from build123d import *

# Parameters (mm, degrees)
SKETCH1_W           = 160
SKETCH1_H           = 90
SKETCH1_R           = 20
SKETCH1_R_2         = 1.5
SKETCH1_W_2         = 10
SKETCH1_H_2         = 3
BOSS_EXTRUDE1_DEPTH = 3


with BuildPart() as part:
    # Sketch1 → Boss-Extrude1 (new body)
    with BuildSketch(Plane(origin=(0, 0, 0), x_dir=(1, 0, 0), z_dir=(0, 1, 0))):
        with Locations((-80, 45)):
            Rectangle(SKETCH1_W, SKETCH1_H)
        with Locations(Location((-40, 50, 0), (0, 0, 270))):
            Circle(SKETCH1_R, mode=Mode.SUBTRACT)
        with Locations(Location((-105, 4, 0), (0, 0, 270))):
            Circle(SKETCH1_R_2, mode=Mode.SUBTRACT)
        with Locations(Location((-45, 4, 0), (0, 0, 270))):
            Circle(SKETCH1_R_2, mode=Mode.SUBTRACT)
        with Locations(Location((-105, 86, 0), (0, 0, 90))):
            Circle(SKETCH1_R_2, mode=Mode.SUBTRACT)
        with Locations(Location((-45, 86, 0), (0, 0, 90))):
            Circle(SKETCH1_R_2, mode=Mode.SUBTRACT)
        with Locations(Location((-140, 67, 0), (0, 0, 270))):
            Circle(SKETCH1_R_2, mode=Mode.SUBTRACT)
        with Locations(Location((-140, 44, 0), (0, 0, 90))):
            Circle(SKETCH1_R_2, mode=Mode.SUBTRACT)
        with Locations(Location((-140, 22, 0), (0, 0, 270))):
            Circle(SKETCH1_R_2, mode=Mode.SUBTRACT)
        Polygon((-118, 68.4), (-118, 31.8), (-90, 31.8), (-80, 41.8), (-68, 41.8), (-61, 45), (-61, 55), (-68, 58.4), (-80, 58.4), (-90, 68.4), align=None, mode=Mode.SUBTRACT)
        with Locations((-135, 84.5)):
            Rectangle(SKETCH1_W_2, SKETCH1_H_2, mode=Mode.SUBTRACT)
        with Locations((-135, 5.5)):
            Rectangle(SKETCH1_W_2, SKETCH1_H_2, mode=Mode.SUBTRACT)
        with Locations((-75, 5.5)):
            Rectangle(SKETCH1_W_2, SKETCH1_H_2, mode=Mode.SUBTRACT)
        with Locations((-75, 84.5)):
            Rectangle(SKETCH1_W_2, SKETCH1_H_2, mode=Mode.SUBTRACT)
        with Locations((-15, 5.5)):
            Rectangle(SKETCH1_W_2, SKETCH1_H_2, mode=Mode.SUBTRACT)
        with Locations((-15, 84.5)):
            Rectangle(SKETCH1_W_2, SKETCH1_H_2, mode=Mode.SUBTRACT)
        with Locations((-151, 67)):
            Rectangle(SKETCH1_W_2, SKETCH1_H_2, mode=Mode.SUBTRACT)
        with Locations((-129, 67)):
            Rectangle(SKETCH1_W_2, SKETCH1_H_2, mode=Mode.SUBTRACT)
        with Locations((-129, 44)):
            Rectangle(SKETCH1_W_2, SKETCH1_H_2, mode=Mode.SUBTRACT)
        with Locations((-151, 44)):
            Rectangle(SKETCH1_W_2, SKETCH1_H_2, mode=Mode.SUBTRACT)
        with Locations((-151, 22)):
            Rectangle(SKETCH1_W_2, SKETCH1_H_2, mode=Mode.SUBTRACT)
        with Locations((-129, 22)):
            Rectangle(SKETCH1_W_2, SKETCH1_H_2, mode=Mode.SUBTRACT)
    extrude(amount=BOSS_EXTRUDE1_DEPTH)


solid = part.part
Work out the finished part from the listing and answer in its coordinate system (mm). A direction names the side the tool comes from. Round coordinates to 2 decimals unless told otherwise and drop trailing zeros. Order: outer loops, then holes, each group sorted by start corner. A loop starts at its lowest first (then second) coordinate and runs counter-clockwise, first axis right, second up. Notation, with made-up numbers: M 27,53 L 50,53 A22 cw 50,74 Z; hole C 34,-21 d7. An arc over 180 degrees is marked long. One line per item, written item: value.
Q1. Find section D-D on x = -23. Write down the section's boundary in (y, z).
Derived:
outline: M 0,-90 L 3,-90 L 3,-60.54 L 0,-60.54 Z; M 0,-39.46 L 3,-39.46 L 3,0 L 0,0 Z
Q2. Find section A-A on x = -105. Write down the section's boundary in (y, z).
Derived:
outline: M 0,-90 L 3,-90 L 3,-87.5 L 0,-87.5 Z; M 0,-84.5 L 3,-84.5 L 3,-68.4 L 0,-68.4 Z; M 0,-31.8 L 3,-31.8 L 3,-5.5 L 0,-5.5 Z; M 0,-2.5 L 3,-2.5 L 3,0 L 0,0 Z
Q3. Find section B-B on z = -22. Write down the section's boundary in (x, y).
Derived:
outline: M -160,0 L -156,0 L -156,3 L -160,3 Z; M -146,0 L -141.5,0 L -141.5,3 L -146,3 Z; M -138.5,0 L -134,0 L -134,3 L -138.5,3 Z; M -124,0 L 0,0 L 0,3 L -124,3 Z
Q4. For faces 1 (the face through (0, 1, -44)), 2 (the face through (-151, 1, -20.5)), determine the directions among +Z, -Z, +X, -X, +Y, -Y from which every point of the face is accessible in a straight line to the end or side of a thin tool.
Derived:
face 1: +Z, -Z, +X, +Y, -Y
face 2: +Y, -Y
Q5. Find section C-C on z = -50. Write down the section's boundary in (x, y), then the cut area to 3 significant figures.
Derived:
outline: M -160,0 L -118,0 L -118,3 L -160,3 Z; M -61,0 L -60,0 L -60,3 L -61,3 Z; M -20,0 L 0,0 L 0,3 L -20,3 Z
area: 189 mm²
Q6. Straight lines are drawn through the part: line 1 (Z direction, x = -137, y = 2.85); line 2 (X direction, y = 0.9, z = -50); line 3 (X direction, y = 2.4, z = -22). For each, find the intervals that lie inside material, in ascending order.
Derived:
line 1: -90 to -86, -83 to -7, -4 to 0
line 2: -160 to -118, -61 to -60, -20 to 0
line 3: -160 to -156, -146 to -141.5, -138.5 to -134, -124 to 0
